The listing builds one solid part. Answer for the finished solid, in the listing's coordinates (mm). Face numbers are marked on the shaded views. A direction names the side the tool comes from. Round coordinates to 2 decimals unless told otherwise and drop trailing zeros. Order: outer loops, then holes, each group sorted by start corner. A loop starts at its lowest first (then second) coordinate and runs counter-clockwise, first axis right, second up. Notation, with made-up numbers: (-7.75, -1.75) - (39.25, -1.75) arc R10 cw to (39.25, 15.25) - close; hole circle Ø10 at (-24, -13.75). An arc over 180 degrees is marked (long way). Use CSV: the item, a comma, the result in double quotes. Start each with the question number.
Item 1: Find section C-C, the plane y = 14.5. Give the vertices of the cut face in (x, z) (3 decimals), plus the area to 3 significant figures.
Item 2: Find section B-B, the plane y = -12. Give the vertices of the cut face in (x, z).
Item 3: Find section A-A, the plane z = 5. Give the vertices of the cut face in (x, y).
Item 4: Flat-ended cylindrical pins translate along their axes: P1, Ø1.5, axis at y = -3, z = 7.5, coming from the +X side; P2, Ø3, axis at x = -4, z = 5, coming from the +Y side; P3, Ø4.5, axis at y = 2, z = 8, coming from the -X side; P4, Ø2, axis at x = -16, z = 5.5, coming from the +Y side. Find the tip coordinate at first contact, or state that the pin passes through.
Item 5: Find section D-D, the plane x = -16. Give the vertices of the cut face in (y, z), plus the area to 3 significant figures.
Item 6: Determine the mould class of the marked faces 1, 2 and 3 for opening direction Z: +Z half, -Z half, draft (parallel to the pull), parting line (faces both ways), or undercut.
Item 7: Straight lines are drawn through the part: line 1 along Y through (x, z) = (-16, 8); line 2 along Y through (x, z) = (-17.5, 4); line 3 along X through (y, z) = (-19.5, 5). For each, find the intervals that lie inside material, in ascending order. Write a range as [from, to].
Item 8: For the marked faces 4, 5 and 6, determine the directions among +Z, -Z, +X, -X, +Y, -Y from which every point of the face is accessible in a straight line to the end or side of a thin tool.
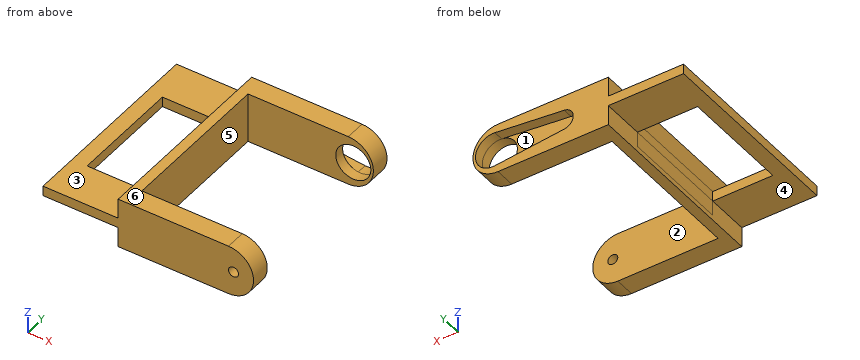
```python
from build123d import *
from build123d.topology import SkipClean

# Parameters (mm, degrees)
BOSS_EXTRUDE1_DEPTH = 10
SKETCH2_W           = 15
SKETCH2_H           = 2
BOSS_EXTRUDE2_DEPTH = 39
FILLET1_RADIUS      = 5
FILLET1_LENGTH      = 4
FILLET2_RADIUS      = 5
FILLET2_LENGTH      = 4
SKETCH6_R           = 1
CUT_EXTRUDE3_DEPTH  = 43
CUT_EXTRUDE4_DEPTH  = 2
SKETCH9_R           = 3.5
CUT_EXTRUDE5_DEPTH  = 8
SKETCH10_W          = 12
SKETCH10_H          = 22
CUT_EXTRUDE6_DEPTH  = 5


with BuildPart() as part:
    # Sketch1 → Boss-Extrude1 (new body)
    with BuildSketch(Plane.XY):
        Polygon((-27, 17.343669269), (0, 17.343669269), (0, 13.343669269), (-25, 13.343669269), (-25, -17.656330731), (0, -17.656330731), (0, -21.656330731), (-27, -21.656330731), align=None)
    extrude(amount=BOSS_EXTRUDE1_DEPTH)

    # Sketch2 → Boss-Extrude2 (add)
    with BuildSketch(Plane(origin=(0, 17.343669269, 0), x_dir=(1, 0, 0), z_dir=(0, 1, 0))):
        with Locations((-34.5, -5)):
            Rectangle(SKETCH2_W, SKETCH2_H)
    extrude(amount=-BOSS_EXTRUDE2_DEPTH)

    # Fillet1: full round fillet: the end face becomes a half cylinder, R = half its width
    fillet1_face = Plane((0, 15.343669269, 5), x_dir=(0, -1, 0), z_dir=(1, 0, 0))  # on the end face: x along it, z out of the body
    fillet1_slab = fillet1_face.offset(-FILLET1_RADIUS / 2) * Box(FILLET1_LENGTH, 2 * FILLET1_RADIUS, FILLET1_RADIUS, mode=Mode.PRIVATE)  # the body's end, R deep
    fillet1_round = Plane((-5, 15.343669269, 5), x_dir=(1, 0, 0), z_dir=(0, -1, 0)) * Cylinder(FILLET1_RADIUS, FILLET1_LENGTH, mode=Mode.PRIVATE)  # its axis R under the face
    add(fillet1_slab - fillet1_round, mode=Mode.SUBTRACT)

    # Fillet2: full round fillet: the end face becomes a half cylinder, R = half its width
    fillet2_face = Plane((0, -19.656330731, 5), x_dir=(0, 1, 0), z_dir=(1, 0, 0))  # on the end face: x along it, z out of the body
    fillet2_slab = fillet2_face.offset(-FILLET2_RADIUS / 2) * Box(FILLET2_LENGTH, 2 * FILLET2_RADIUS, FILLET2_RADIUS, mode=Mode.PRIVATE)  # the body's end, R deep
    fillet2_round = Plane((-5, -19.656330731, 5), x_dir=(1, 0, 0), z_dir=(0, 1, 0)) * Cylinder(FILLET2_RADIUS, FILLET2_LENGTH, mode=Mode.PRIVATE)  # its axis R under the face
    add(fillet2_slab - fillet2_round, mode=Mode.SUBTRACT)

    # Sketch6 → Cut-Extrude3 (cut)
    with BuildSketch(Plane(origin=(0, 17.343669269, 0), x_dir=(1, 0, 0), z_dir=(0, 1, 0))):
        with Locations(Location((-4, -5, 0), (0, 0, 270))):
            Circle(SKETCH6_R)
    extrude(amount=-CUT_EXTRUDE3_DEPTH, mode=Mode.SUBTRACT)

    # Sketch8 → Cut-Extrude4 (cut)
    with BuildSketch(Plane(origin=(0, 17.343669269, 0), x_dir=(1, 0, 0), z_dir=(0, 1, 0))):
        with BuildLine():
            Line((-18.214285714, -3.011512728), (-4.375, -1.520147273))
            ThreePointArc((-4.375, -1.520147273), (-0.5, -5), (-4.375, -8.479852727))
            Line((-4.375, -8.479852727), (-18.214285714, -6.988487272))
            ThreePointArc((-18.214285714, -6.988487272), (-20, -5), (-18.214285714, -3.011512728))
        make_face()
    extrude(amount=-CUT_EXTRUDE4_DEPTH, mode=Mode.SUBTRACT)

    # Sketch9 → Cut-Extrude5 (cut)
    with SkipClean():  # the faces are left unmerged after this step: merging them gives an invalid solid
        with BuildSketch(Plane(origin=(0, 17.343669269, 0), x_dir=(1, 0, 0), z_dir=(0, 1, 0))):
            with Locations(Location((-4, -5, 0), (0, 0, 263.849360172))):
                Circle(SKETCH9_R)
        extrude(amount=-CUT_EXTRUDE5_DEPTH, mode=Mode.SUBTRACT)

    # Sketch10 → Cut-Extrude6 (cut)
    with SkipClean():  # the faces are left unmerged after this step: merging them gives an invalid solid
        with BuildSketch(Plane.XY.offset(6)):
            with Locations((-33, -2.156330731)):
                Rectangle(SKETCH10_W, SKETCH10_H)
        extrude(amount=-CUT_EXTRUDE6_DEPTH, mode=Mode.SUBTRACT)


solid = part.part
```
Worked out:
1,outline,"(-42, 4) - (-27, 4) - (-27, 0) - (-5, 0) arc R5 ccw to (-5, 10) - (-27, 10) - (-27, 6) - (-42, 6) - close; hole circle Ø7 at (-4, 5)"
1,area,"251 mm²"
2,outline,"(-42, 4) - (-39, 4) - (-39, 6) - (-42, 6) - close; (-27, 0) - (-25, 0) - (-25, 10) - (-27, 10) - close"
3,outline,"(-42, -21.66) - (-5, -21.66) - (-5, -17.66) - (-25, -17.66) - (-25, 13.34) - (-7.5, 13.34) - (-7.5, 15.34) - (-20, 15.34) - (-20, 17.34) - (-42, 17.34) - close; (-3, -21.66) - (0, -21.66) - (0, -17.66) - (-3, -17.66) - close; (-0.5, 13.34) - (0, 13.34) - (0, 17.34) - (-0.5, 17.34) - close; hole (-39, -13.16) - (-27, -13.16) - (-27, 8.84) - (-39, 8.84) - close"
4,P1,"stops at x = -25"
4,P2,"stops at y = -17.66"
4,P3,"stops at x = -42"
4,P4,"stops at y = 15.34"
5,outline,"(-21.66, 0) - (-17.66, 0) - (-17.66, 10) - (-21.66, 10) - close; (13.34, 0) - (17.34, 0) - (17.34, 2.77) - (15.34, 2.77) - (15.34, 7.23) - (17.34, 7.23) - (17.34, 10) - (13.34, 10) - close"
5,area,"71.1 mm²"
6,face 1,"undercut"
6,face 2,"draft"
6,face 3,"+Z half"
7,line 1,"y = [-21.66, -17.66], [13.34, 17.34]"
7,line 2,"y = [-21.66, -17.66], [13.34, 15.34]"
7,line 3,"x = [-42, -5], [-3, 0]"
8,face 4,"-Z, -X, +Y, -Y"
8,face 5,"+Z, -Z, +X"
8,face 6,"+Z, +X, -X, +Y, -Y"
